```python
from build123d import *

# Parameters (mm, degrees)
F1_DEPTH    = 2.5
F2_T1_DEPTH = 14.9498743711
F2_T3_DEPTH = 15


# Not quite as in the source:
# - a fillet or chamfer that OpenCascade refuses, or shapes differently, is made with other operations: its cross-section is extruded or revolved along the edge and cut away or added


with BuildPart() as f1:
    # F0 (on Top) → F1 (new body, symmetric)
    with BuildSketch(Plane.XY):
        Polygon((1.8475208614, 3.2), (3.6950417228, 0), (1.8475208614, -3.2), (-1.8475208614, -3.2), (-1.8475208614, -5), (5.1524791386, -5), (9.4826061575, -2.5), (58.1524791386, -2.5), (58.1524791386, 2.5), (9.4826061575, 2.5), (5.1524791386, 5), (-1.8475208614, 5), (-1.8475208614, 3.2), align=None)
    extrude(amount=F1_DEPTH, both=True)

    # F2: fillet of radius 2 on 4 edges, made by hand

    # F2_s2 → F2_t1 (cut)
    with BuildSketch(Plane.XY.offset(-7.4749371855)):
        with BuildLine():
            ThreePointArc((-1.8475208614, 5), (-1.1991867737, 3.7167603026), (0.1424540128, 3.2))
            Line((0.1424540128, 3.2), (-1.8475208614, 3.2))
            Line((-1.8475208614, 3.2), (-1.8475208614, 5))
        make_face()
        with BuildLine():
            ThreePointArc((-1.8475208614, -5), (-1.1991867737, -3.7167603026), (0.1424540128, -3.2))
            Line((0.1424540128, -3.2), (-1.8475208614, -3.2))
            Line((-1.8475208614, -3.2), (-1.8475208614, -5))
        make_face()
    extrude(amount=F2_T1_DEPTH, mode=Mode.SUBTRACT)

    # F2_s4 → F2_t3 (cut)
    with BuildSketch(Plane.XY.offset(-7.5)):
        with BuildLine():
            ThreePointArc((58.1524791386, -0.5), (57.566692701, -1.9142135624), (56.1524791386, -2.5))
            Line((56.1524791386, -2.5), (58.1524791386, -2.5))
            Line((58.1524791386, -2.5), (58.1524791386, -0.5))
        make_face()
        with BuildLine():
            ThreePointArc((56.1524791386, 2.5), (57.566692701, 1.9142135624), (58.1524791386, 0.5))
            Line((58.1524791386, 0.5), (58.1524791386, 2.5))
            Line((58.1524791386, 2.5), (56.1524791386, 2.5))
        make_face()
    extrude(amount=F2_T3_DEPTH, mode=Mode.SUBTRACT)


solid = f1.part
```
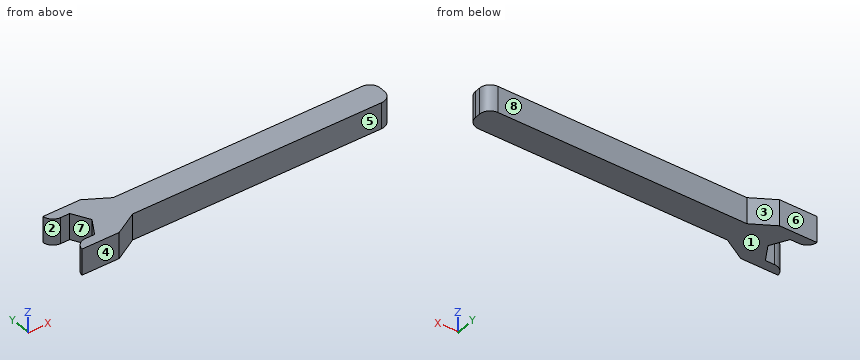
Build history of the part. All positions in model axes, mm. Face numbers are marked on the shaded views. A direction names the side the tool comes from. Give positions to 0.01 mm unless a question says otherwise; leave off trailing zeros. Loops run counter-clockwise (first coordinate to the right, second up) from the corner with the lowest first, then second, coordinate; pieces in that order, holes last. Notation, with made-up numbers: (-4, 36) -> (9, 36) arc R13 cw to (9, 49) -> close; hole circle Ø4 at (67, -22.5). An arc over 180 degrees is marked (long way). One line per question, with ' | ' between items. Start each with the question number.
1) Cut at C-C (x = 36.5). Give the cut face in (y, z).
2) Pin check, flat tips, straight feed: pin 1 (2.5 mm diameter, centred on x = 28, z = 1, fed in from -Y); pin 2 (3 mm diameter, centred on y = -1, z = 1, fed in from -X); pin 3 (1.5 mm diameter, centred on x = 12.5, z = -0.5, fed in from +Y). Stop position of each tip, or through.
3) Cut at B-B (y = -2). Give the cut face in (x, z).
4) Cut at A-A (z = 1.35). Give the cut face in (x, y).
5) 3-axis set-ups, long thin cutter, end or side, ignore diameter. For the marked faces 4, 5, 6, 7 and 8: which of +Z, -Z, +X, -X, +Y, -Y reach the whole face in a straight line?
6) Probe L1, parallel to Y at x = 26, z = 0.1; L2, parallel to X at y = 0.5, z = 0.35; L3, parallel to X at y = 2.75, z = 0.85. List the from-to ranges inside material, lowest first.
7) Two-plate mould, pull along X, no slides. Class the marked faces 1, 2 and 3: released by +X, released by -X, zero draft, split by the parting line, or undercut.
Return value:
1) outline: (-2.5, -2.5) -> (2.5, -2.5) -> (2.5, 2.5) -> (-2.5, 2.5) -> close
2) pin 1: y = -2.5 | pin 2: x = 2.25 | pin 3: y = 2.5
3) outline: (2.54, -2.5) -> (57.48, -2.5) -> (57.48, 2.5) -> (2.54, 2.5) -> close
4) outline: (-1.85, -5) -> (5.15, -5) -> (9.48, -2.5) -> (56.15, -2.5) arc R2 ccw to (58.15, -0.5) -> (58.15, 0.5) arc R2 ccw to (56.15, 2.5) -> (9.48, 2.5) -> (5.15, 5) -> (-1.85, 5) arc R2 ccw to (0.14, 3.2) -> (1.85, 3.2) -> (3.7, 0) -> (1.85, -3.2) -> (0.14, -3.2) arc R2 ccw to start
5) face 4: +Z, -Z, +X, -X, -Y | face 5: +Z, -Z, +X, -Y | face 6: +Z, -Z, +X, -X, +Y | face 7: +Z, -Z, -X | face 8: +Z, -Z, +X, +Y
6) L1: -2.5 to 2.5 | L2: 3.41 to 58.15 | L3: 2.11 to 9.05
7) face 1: zero draft | face 2: released by -X | face 3: released by +X
